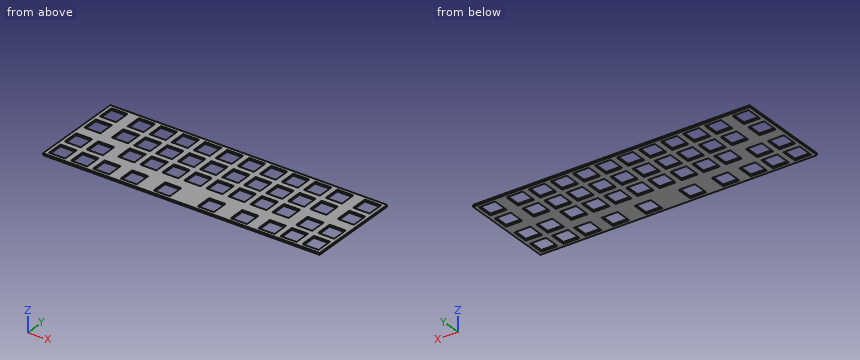
```python
from build123d import *

# Parameters (mm, degrees)
SKETCH036_W     = 119.5625
SKETCH036_H     = 81.9625
PAD015_DEPTH    = 1.6
SKETCH037_W     = 14
SKETCH037_H     = 14
POCKET022_DEPTH = 5
SKETCH038_W     = 14
SKETCH038_H     = 14
POCKET023_DEPTH = 5
SKETCH039_W     = 14
SKETCH039_H     = 14
POCKET024_DEPTH = 5


with BuildPart() as plate:
    # Sketch036 → Pad015 (new body)
    with BuildSketch(Plane.XY):
        with Locations((-59.78125, 0)):
            Rectangle(SKETCH036_W, SKETCH036_H)
    extrude(amount=-PAD015_DEPTH)

    # Sketch037 → Pocket022 (cut)
    with BuildSketch(Plane.XY):
        with Locations((-9.525, 30.98125)):
            Rectangle(SKETCH037_W, SKETCH037_H)
        with Locations((-28.575, 30.98125)):
            Rectangle(SKETCH037_W, SKETCH037_H)
        with Locations((-47.625, 30.98125)):
            Rectangle(SKETCH037_W, SKETCH037_H)
        with Locations((-66.675, 30.98125)):
            Rectangle(SKETCH037_W, SKETCH037_H)
        with Locations((-85.725, 30.98125)):
            Rectangle(SKETCH037_W, SKETCH037_H)
        with Locations((-85.725, 11.93125)):
            Rectangle(SKETCH037_W, SKETCH037_H)
        with Locations((-66.675, 11.93125)):
            Rectangle(SKETCH037_W, SKETCH037_H)
        with Locations((-9.525, 11.93125)):
            Rectangle(SKETCH037_W, SKETCH037_H)
        with Locations((-47.625, 11.93125)):
            Rectangle(SKETCH037_W, SKETCH037_H)
        with Locations((-28.575, 11.93125)):
            Rectangle(SKETCH037_W, SKETCH037_H)
        with Locations((-9.525, -7.11875)):
            Rectangle(SKETCH037_W, SKETCH037_H)
        with Locations((-28.575, -7.11875)):
            Rectangle(SKETCH037_W, SKETCH037_H)
        with Locations((-47.625, -7.11875)):
            Rectangle(SKETCH037_W, SKETCH037_H)
        with Locations((-66.675, -7.11875)):
            Rectangle(SKETCH037_W, SKETCH037_H)
    extrude(amount=-POCKET022_DEPTH, mode=Mode.SUBTRACT)

    # Sketch038 → Pocket023 (cut)
    with BuildSketch(Plane.XY):
        with Locations((-109.5625, 30.98125)):
            Rectangle(SKETCH038_W, SKETCH038_H)
        with Locations((-109.5625, 11.93125)):
            Rectangle(SKETCH038_W, SKETCH038_H)
        with Locations((-109.5625, -11.93125)):
            Rectangle(SKETCH038_W, SKETCH038_H)
        with Locations((-109.5625, -30.98125)):
            Rectangle(SKETCH038_W, SKETCH038_H)
        with Locations((-90.5125, -11.93125)):
            Rectangle(SKETCH038_W, SKETCH038_H)
        with Locations((-90.5125, -30.98125)):
            Rectangle(SKETCH038_W, SKETCH038_H)
        with Locations((-71.4625, -30.98125)):
            Rectangle(SKETCH038_W, SKETCH038_H)
    extrude(amount=-POCKET023_DEPTH, mode=Mode.SUBTRACT)

    # Sketch039 → Pocket024 (cut)
    with BuildSketch(Plane.XY):
        with Locations((-47.625, -30.98125)):
            Rectangle(SKETCH039_W, SKETCH039_H)
        with Locations((-19.05, -30.98125)):
            Rectangle(SKETCH039_W, SKETCH039_H)
    extrude(amount=-POCKET024_DEPTH, mode=Mode.SUBTRACT)


with BuildPart() as case_plate:
    # Part__Mirroring002: instance of plate
    add(plate.part.mirror(Plane(origin=(0, 0, 0), x_dir=(0, -1, 0), z_dir=(1, 0, 0))))

    # Fusion002: union plate
    add(plate.part)


solid = case_plate.part
```
Design review of the part built by this model. Coordinates are the model's own, in mm. Give positions to 0.01 mm unless a question says otherwise; leave off trailing zeros. Write each loop counter-clockwise with the first axis right and the second up, starting at its lowest first coordinate (ties: lowest second). Pieces come first, ordered by that corner, then holes.
(1) Add section A-A (x = 32). Give the boundary of the cut face in (y, z).
Checked values:
outline: (-40.98, -1.6) - (-14.12, -1.6) - (-14.12, 0) - (-40.98, 0) - close; (-0.12, -1.6) - (4.93, -1.6) - (4.93, 0) - (-0.12, 0) - close; (18.93, -1.6) - (23.98, -1.6) - (23.98, 0) - (18.93, 0) - close; (37.98, -1.6) - (40.98, -1.6) - (40.98, 0) - (37.98, 0) - close
(2) Wall thickness on line 1 along Y through (x, z) = (30, -0.4); line 2 along Y through (x, z) = (-87, -0.75); line 3 along Y through (x, z) = (-41.5, -1.25): over which ranges is each line inside the solid? List them lowest first.
Checked values:
line 1: y = -40.98 to -14.12, -0.12 to 4.93, 18.93 to 23.98, 37.98 to 40.98
line 2: y = -40.98 to -37.98, -23.98 to -18.93, -4.93 to 4.93, 18.93 to 23.98, 37.98 to 40.98
line 3: y = -40.98 to -37.98, -23.98 to -14.12, -0.12 to 4.93, 18.93 to 23.98, 37.98 to 40.98
(3) Add section B-B (y = -32). Give the number of separate pieces and of enclosed holes in the cut face, and give its area (3 significant figures).
Checked values:
separate pieces: 11
enclosed holes: 0
area: 159 mm2
